from build123d import *

# Parameters (mm, degrees)
SKETCH1_W           = 150
SKETCH1_H           = 150
SKETCH1_W_2         = 140
SKETCH1_H_2         = 140
BOSS_EXTRUDE1_DEPTH = 20
SKETCH1_3_W         = 140
SKETCH1_3_H         = 140
SKETCH1_3_R         = 2
BOSS_EXTRUDE2_DEPTH = 10
SKETCH1_4_R         = 57.5
CUT_EXTRUDE1_DEPTH  = 4
SKETCH1_5_R         = 2.9
CUT_EXTRUDE2_DEPTH  = 10


with BuildPart() as part:
    # Sketch1 → Boss-Extrude1 (new body)
    with BuildSketch(Plane(origin=(0, 0, 0), x_dir=(1, 0, 0), z_dir=(0, 1, 0))):
        Rectangle(SKETCH1_W, SKETCH1_H)
        Rectangle(SKETCH1_W_2, SKETCH1_H_2, mode=Mode.SUBTRACT)
    extrude(amount=BOSS_EXTRUDE1_DEPTH)

    # Sketch1<3> → Boss-Extrude2 (add)
    with BuildSketch(Plane(origin=(0, 0, 0), x_dir=(1, 0, 0), z_dir=(0, 1, 0))):
        Rectangle(SKETCH1_3_W, SKETCH1_3_H)
        with Locations(Location((-62.1, -62.1, 0), (0, 0, 270))):
            Circle(SKETCH1_3_R, mode=Mode.SUBTRACT)
        with Locations(Location((62.1, -62.1, 0), (0, 0, 270))):
            Circle(SKETCH1_3_R, mode=Mode.SUBTRACT)
        with Locations(Location((-62.1, 62.1, 0), (0, 0, 270))):
            Circle(SKETCH1_3_R, mode=Mode.SUBTRACT)
        with Locations(Location((62.1, 62.1, 0), (0, 0, 270))):
            Circle(SKETCH1_3_R, mode=Mode.SUBTRACT)
    extrude(amount=BOSS_EXTRUDE2_DEPTH)

    # Sketch1<4> → Cut-Extrude1 (cut)
    with BuildSketch(Plane(origin=(0, 0, 0), x_dir=(1, 0, 0), z_dir=(0, 1, 0))):
        with Locations(Location((0, 0, 0), (0, 0, 270))):
            Circle(SKETCH1_4_R)
    extrude(amount=CUT_EXTRUDE1_DEPTH, mode=Mode.SUBTRACT)

    # Sketch1<5> → Cut-Extrude2 (cut)
    with BuildSketch(Plane(origin=(0, 0, 0), x_dir=(1, 0, 0), z_dir=(0, 1, 0))):
        with Locations(Location((0, 0, 0), (0, 0, 270))):
            Circle(SKETCH1_5_R)
    extrude(amount=CUT_EXTRUDE2_DEPTH, mode=Mode.SUBTRACT)


solid = part.part
Check sheet for the modelled part. Datum: model origin and axes. Units: mm. A direction names the side the tool comes from. Coordinates: 2 decimals unless noted, no trailing zeros. Loops run counter-clockwise (first coordinate to the right, second up) from the corner with the lowest first, then second, coordinate; pieces in that order, holes last. Notation, with made-up numbers: (61.5, 87.5) -> (96.5, 87.5) arc R26 ccw to (96.5, 102.5) -> close; hole circle Ø6 at (11, -35.75). An arc over 180 degrees is marked (long way). Write item = value, one per line. Start each with the question number.
1. Section check D-D on y = 17.5. Record the cut outline in (x, z), then the cut area to 3 significant figures.
2. Tool access check on faces 4 (the flat face through (1, 4, 12)), 5 (the flat face through (-75, 10, 1)), 6 (the flat face through (15, 10, -1)). Record the directions out of +Z, -Z, +X, -X, +Y, -Y that give a thin tool (end or side, any length) a straight path to the whole face; none if there is none.
3. Section check C-C on z = -62.1. Record the cut outline in (x, y).
4. Depth check by flat-ended pin: P1, Ø5, axis at x = 62.1, z = -62.1, coming from the +Y side; P2, Ø9.5, axis at x = 0, z = 0, coming from the -Y side. Enter the tip coordinate at first touch or a pass-through.
5. Section check B-B on z = 0. Record the cut outline in (x, y).
6. Draft check along X on faces 1 (the flat face through (75, 10, 1)), 2 (the cylindrical face through (-63.3, 4.9, 60.5)), 3 (the flat face through (-1, 10, 75)). Enter one of: released by +X, released by -X, zero draft, split by the parting line, or undercut.
7. Section check A-A on x = 0. Record the cut outline in (y, z).
8. Material ranges on line 1 (X direction, y = 6.45, z = 0); line 2 (X direction, y = 13, z = -29.5); line 3 (X direction, y = 6.5, z = -62.1), recorded low to high.
Responses:
q1.outline = (-75, -75) -> (75, -75) -> (75, 75) -> (-75, 75) -> close; hole (-70, -70) -> (70, -70) -> (70, 70) -> (-70, 70) -> close
q1.area = 2,900 mm2
q2.face_4 = -Y
q2.face_5 = +Z, -Z, -X, +Y, -Y
q2.face_6 = +Y
q3.outline = (-75, 0) -> (-64.1, 0) -> (-64.1, 10) -> (-70, 10) -> (-70, 20) -> (-75, 20) -> close; (-60.1, 0) -> (60.1, 0) -> (60.1, 10) -> (-60.1, 10) -> close; (64.1, 0) -> (75, 0) -> (75, 20) -> (70, 20) -> (70, 10) -> (64.1, 10) -> close
q4.P1 = 10
q4.P2 = 4
q5.outline = (-75, 0) -> (-57.5, 0) -> (-57.5, 4) -> (-2.9, 4) -> (-2.9, 10) -> (-70, 10) -> (-70, 20) -> (-75, 20) -> close; (2.9, 4) -> (57.5, 4) -> (57.5, 0) -> (75, 0) -> (75, 20) -> (70, 20) -> (70, 10) -> (2.9, 10) -> close
q6.face_1 = released by +X
q6.face_2 = undercut
q6.face_3 = zero draft
q7.outline = (0, -75) -> (20, -75) -> (20, -70) -> (10, -70) -> (10, -2.9) -> (4, -2.9) -> (4, -57.5) -> (0, -57.5) -> close; (0, 57.5) -> (4, 57.5) -> (4, 2.9) -> (10, 2.9) -> (10, 70) -> (20, 70) -> (20, 75) -> (0, 75) -> close
q8.line_1 = -75 to -2.9, 2.9 to 75
q8.line_2 = -75 to -70, 70 to 75
q8.line_3 = -75 to -64.1, -60.1 to 60.1, 64.1 to 75
